from build123d import *

# Parameters (mm, degrees)
BOSS_EXTRUDE1_DEPTH = 120
BOSS_EXTRUDE2_DEPTH = 10
BOSS_EXTRUDE3_START = 120
BOSS_EXTRUDE3_DEPTH = 10
FILLET1_R           = 5
FILLET2_R           = 15
FILLET3_R           = 2
FILLET4_R           = 4


with BuildPart() as part:
    # Sketch1 → Boss-Extrude1 (new body)
    with BuildSketch(Plane(origin=(0, 0, 0), x_dir=(1, 0, 0), z_dir=(0, 1, 0))):
        Polygon((-15.2, -55.784127273), (-15.2, -65), (-10.2, -65), (-10.2, -20.4), (-10.2, 0), (10.2, 0), (10.2, -20.4), (10.2, -65), (15.2, -65), (15.2, -55.784127273), (15.2, -9.142135624), (15.2, 5), (-15.2, 5), (-15.2, -9.142135624), align=None)
    extrude(amount=BOSS_EXTRUDE1_DEPTH)

    # Sketch1<3> → Boss-Extrude2 (add)
    with BuildSketch(Plane(origin=(0, 0, 0), x_dir=(1, 0, 0), z_dir=(0, 1, 0))):
        Polygon((-110, 99.8), (-117.071067812, 92.728932188), (-100.263572466, 75.921436842), (-15.2, -9.142135624), (-15.2, 5), align=None)
        Polygon((110, 99.8), (15.2, 5), (15.2, -9.142135624), (100.263572466, 75.921436842), (117.071067812, 92.728932188), align=None)
        Polygon((100.263572466, 75.921436842), (15.2, -55.784127273), (15.2, -65), (117.071067812, 92.728932188), align=None)
        Polygon((-100.263572466, 75.921436842), (-117.071067812, 92.728932188), (-15.2, -65), (-15.2, -55.784127273), align=None)
    extrude(amount=BOSS_EXTRUDE2_DEPTH)

    # Sketch1<4> → Boss-Extrude3 (add)
    with BuildSketch(Plane(origin=(0, 0, 0), x_dir=(1, 0, 0), z_dir=(0, 1, 0)).offset(BOSS_EXTRUDE3_START)):
        Polygon((-110, 99.8), (-117.071067812, 92.728932188), (-100.263572466, 75.921436842), (-15.2, -9.142135624), (-15.2, 5), align=None)
        Polygon((-100.263572466, 75.921436842), (-117.071067812, 92.728932188), (-15.2, -65), (-15.2, -55.784127273), align=None)
        Polygon((110, 99.8), (15.2, 5), (15.2, -9.142135624), (100.263572466, 75.921436842), (117.071067812, 92.728932188), align=None)
        Polygon((100.263572466, 75.921436842), (15.2, -55.784127273), (15.2, -65), (117.071067812, 92.728932188), align=None)
    extrude(amount=-BOSS_EXTRUDE3_DEPTH)

    # Fillet1
    fillet1_edges = [part.edges().sort_by_distance(p)[0] for p in [
        (15.2, 5, 9.142135624),
        (100.263572466, 5, -75.921436842),
        (15.2, 5, 55.784127273),
        (-15.2, 5, 55.784127273),
        (-100.263572466, 5, -75.921436842),
        (-15.2, 5, 9.142135624),
        (-100.263572466, 115, -75.921436842),
        (-15.2, 115, 55.784127273),
        (-15.2, 115, 9.142135624),
        (15.2, 115, 55.784127273),
        (100.263572466, 115, -75.921436842),
        (15.2, 115, 9.142135624),
    ]]
    fillet(fillet1_edges, radius=FILLET1_R)

    # Fillet2
    fillet2_edges = [part.edges().sort_by_distance(p)[0] for p in [
        (-15.2, 115, -5),
        (15.2, 115, -5),
        (15.2, 5, -5),
        (-15.2, 5, -5),
    ]]
    fillet(fillet2_edges, radius=FILLET2_R)

    # Fillet3
    fillet3_edges = [part.edges().sort_by_distance(p)[0] for p in [
        (10.2, 60, 0),
        (-10.2, 60, 0),
    ]]
    fillet(fillet3_edges, radius=FILLET3_R)

    # Fillet4
    fillet4_edges = [part.edges().sort_by_distance(p)[0] for p in [
        (117.071067812, 5, -92.728932188),
        (110, 5, -99.8),
        (-110, 5, -99.8),
        (-117.071067812, 5, -92.728932188),
        (-117.071067812, 115, -92.728932188),
        (-110, 115, -99.8),
        (110, 115, -99.8),
        (117.071067812, 115, -92.728932188),
    ]]
    fillet(fillet4_edges, radius=FILLET4_R)


solid = part.part
Can you work these out from the model? Positions are in its coordinate system, mm. A direction names the side the tool comes from. Give positions to 0.01 mm unless a question says otherwise; leave off trailing zeros. Order: outer loops, then holes, each group sorted by start corner. A loop starts at its lowest first (then second) coordinate and runs counter-clockwise, first axis right, second up. Notation, with made-up numbers: M 81,55 L 136,55 A36 cw 136,89 Z; hole C 22,22.25 d5. An arc over 180 degrees is marked long. Use one line per item in the form item = value. Start each with the question number.
Item 1: We'd pull the mould along Y, two halves only. Please class faces 1 (the flat face through (62, 110, -41)), 2 (the flat face through (13, 59, 65)): +Y half, -Y half, draft (parallel to the pull), parting line (faces both ways), or undercut.
Item 2: If I drill on line 1 along X through (y, z) = (11.5, 50); line 2 along X through (y, z) = (5, -43.5); line 3 along Z through (x, y) = (12, 82), over which ranges is the centre line in solid material (lowest first)?
Item 3: If we section it at C-C (z = -83.5): Write out the boundary of the cut face in (x, y).
Item 4: If we section it at B-B (x = 83): Write out the boundary of the cut face in (y, z), then the cut area to 3 significant figures.
Item 5: If we section it at A-A (y = 73): Write out the boundary of the cut face in (x, z).
Item 6: Will these pins go through, and if not, where does the flat tip stop? pin 1 Ø1 at (y, z) = (90.5, 38.5) entering from -X; pin 2 Ø21 at (y, z) = (40, 43.5) entering from +X; pin 3 Ø24.5 at (x, y) = (-3.5, 50.5) entering from -Z; pin 4 Ø3 at (x, z) = (-8.5, 16) entering from -Y.
Item 7: If we section it at D-D (z = -31.5): State how many separate pieces and enclosed holes the cut face has, then the cut area to 3 significant figures.
Item 8: For faces 3 (the flat face through (-13, 59, 65)), 4 (the flat face through (49.93, 115.07, 2.01)), 5 (the cylindrical face through (-14.803, 5.07, -6.174)), 6 (the cylindrical face through (115.94, 114.93, -92.57)), 7 (the flat face through (10.2, 59, 33)), which set-ups out of +Z, -Z, +X, -X, +Y, -Y let a thin tool reach every point of the face, with its end or its side?
Outcome:
q1.face_1 = undercut
q1.face_2 = draft
q2.line_1 = -15.2 to -10.2, 10.2 to 15.2
q2.line_2 = -85.28 to -73.02, -68.1 to -53.7, 53.7 to 68.1, 73.02 to 85.28
q2.line_3 = -5 to 65
q3.outline = M -111.11,0 L -93.7,0 L -93.7,10 L -111.11,10 Z; M -111.11,110 L -93.7,110 L -93.7,120 L -111.11,120 Z; M 93.7,0 L 111.11,0 L 111.11,10 L 93.7,10 Z; M 93.7,110 L 111.11,110 L 111.11,120 L 93.7,120 Z
q4.outline = M 0,-72.8 L 10,-72.8 L 10,-39.98 L 0,-39.98 Z; M 110,-72.8 L 120,-72.8 L 120,-39.98 L 110,-39.98 Z
q4.area = 656 mm2
q5.outline = M -15.2,-5 L 15.2,-5 L 15.2,65 L 10.2,65 L 10.2,2 A2 cw 8.2,0 L -8.2,0 A2 cw -10.2,2 L -10.2,65 L -15.2,65 Z
q6.pin_1 = -15.2
q6.pin_2 = 15.2
q6.pin_3 = -5
q6.pin_4 = through
q7.separate_pieces = 8
q7.enclosed_holes = 0
q7.area = 804 mm2
q8.face_3 = +Z, +X, -X, +Y, -Y
q8.face_4 = +Y, -Y
q8.face_5 = -Z, +Y, -Y
q8.face_6 = +X, +Y, -Y
q8.face_7 = +Z, +Y, -Y
